Here's how the part is built. I have some questions about the finished solid (model axes, mm). A direction names the side the tool comes from. Coordinates: 2 decimals unless noted, no trailing zeros. Write each loop counter-clockwise with the first axis right and the second up, starting at its lowest first coordinate (ties: lowest second). Pieces come first, ordered by that corner, then holes.
from build123d import *

# Parameters (mm, degrees)
SKETCH1_R                = 13.7
BOSS_EXTRUDE1_DEPTH      = 101
SKETCH5_W                = 55.5
SKETCH5_H                = 56.561345004
BOSS_EXTRUDE2_DEPTH      = 2.6
CUT_EXTRUDE4_DEPTH       = 2.6
BOSS_EXTRUDE4_DEPTH      = 6
SKETCH8_W                = 33.3
SKETCH8_H                = 11.7
BOSS_EXTRUDE5_DEPTH      = 2.8
SKETCH9_W                = 33.3
SKETCH9_H                = 2.7
BOSS_EXTRUDE6_DEPTH      = 22.2
FILLET2_R                = 5
REVOLVE1_ANGLE           = 40
REVOLVE1_OTHER_WAY_ANGLE = 40
FILLET6_R                = 9


with BuildPart() as part:
    # Sketch1 → Boss-Extrude1 (new body)
    with BuildSketch(Plane.XY):
        with Locations(Location((0, 0, 0), (0, 0, 180))):
            Circle(SKETCH1_R)
    extrude(amount=BOSS_EXTRUDE1_DEPTH)

    # Sketch5 → Boss-Extrude2 (add)
    with BuildSketch(Plane(origin=(0, 0, 0), x_dir=(-1, 0, 0), z_dir=(0, 0, -1))):
        Rectangle(SKETCH5_W, SKETCH5_H)
    extrude(amount=BOSS_EXTRUDE2_DEPTH)

    # Sketch6 → Cut-Extrude4 (cut)
    with BuildSketch(Plane(origin=(0, 0, -2.6), x_dir=(-1, 0, 0), z_dir=(0, 0, -1))):
        Polygon((27.75, 28.280672502), (18.35, 28.280672502), (27.75, 16.680672502), align=None)
        Polygon((-16.15, -28.280672502), (-27.75, -16.680672502), (-27.75, -28.280672502), align=None)
        Polygon((27.75, -18.880672502), (18.35, -28.280672502), (27.75, -28.280672502), align=None)
        Polygon((-27.75, 16.680672502), (-27.75, 28.280672502), (-16.15, 28.280672502), align=None)
    extrude(amount=-CUT_EXTRUDE4_DEPTH, mode=Mode.SUBTRACT)

    # Sketch7 → Boss-Extrude4 (add)
    with BuildSketch(Plane(origin=(0, 0, -2.6), x_dir=(-1, 0, 0), z_dir=(0, 0, -1))):
        Polygon((1.1, 25.680672502), (16.366645995, 25.680672502), (16.366645995, 22.680672502), (-16.933354005, 22.680672502), (-16.933354005, 25.680672502), align=None)
    extrude(amount=BOSS_EXTRUDE4_DEPTH)

    # Sketch8 → Boss-Extrude5 (add)
    with BuildSketch(Plane(origin=(0, 0, -8.6), x_dir=(-1, 0, 0), z_dir=(0, 0, -1))):
        with Locations((-0.283354005, 19.830672502)):
            Rectangle(SKETCH8_W, SKETCH8_H)
    extrude(amount=BOSS_EXTRUDE5_DEPTH)

    # Sketch9 → Boss-Extrude6 (add)
    with BuildSketch(Plane(origin=(0, 25.680672502, 0), x_dir=(1, 0, 0), z_dir=(0, 1, 0))):
        with Locations((0.283354005, 10.05)):
            Rectangle(SKETCH9_W, SKETCH9_H)
    extrude(amount=BOSS_EXTRUDE6_DEPTH)

    # Fillet2
    # the kernel refuses this fillet: 5 mm, written as the material it adds along each edge
    with BuildSketch(Plane(origin=(-16.366645995, 25.680672502, -2.6), x_dir=(0, 1, 0), z_dir=(1, 0, 0))) as fillet2_piece_1_section:
        with BuildLine():
            CenterArc((5, -4.38634244), FILLET2_R, 118.685402014, 61.314597986)
            Line((0, -4.38634244), (-0.1, -4.38634244))
            Line((-0.1, -4.38634244), (-0.1, 0))
            Line((-0.1, 0), (0, 0.1))
            ThreePointArc((0, 0.1), (1.3, 0.1), (2.552, 0.087726849))
            Line((2.552, 0.087726849), (2.6, 0))
        make_face()
    fillet2_piece_1 = extrude(amount=33.3, mode=Mode.PRIVATE)
    fillet2_piece_1 = split(fillet2_piece_1, bisect_by=Plane(origin=(9.175527955, 35.255144547, -3.690317045), z_dir=(-0.7071067811865442, -0.7071067811865509, 0)), keep=Keep.TOP, mode=Mode.PRIVATE)
    add(fillet2_piece_1)
    with BuildSketch(Plane(origin=(-16.366645995, 22.680672502, -2.6), x_dir=(0, -1, 0), z_dir=(1, 0, 0))) as fillet2_piece_2:
        with BuildLine():
            CenterArc((FILLET2_R, FILLET2_R), FILLET2_R, 180, 90)
            Line((0, FILLET2_R), (-FILLET2_R * 0.02, FILLET2_R))
            Line((-FILLET2_R * 0.02, FILLET2_R), (-FILLET2_R * 0.02, -FILLET2_R * 0.02))
            Line((-FILLET2_R * 0.02, -FILLET2_R * 0.02), (FILLET2_R, -FILLET2_R * 0.02))
            Line((FILLET2_R, -FILLET2_R * 0.02), (FILLET2_R, 0))
        make_face()
    extrude(amount=33.3)
    with BuildSketch(Plane(origin=(-16.366645995, 22.680672502, -8.6), x_dir=(0, -1, 0), z_dir=(1, 0, 0)), Plane(origin=(16.933354005, 25.680672502, -8.7), x_dir=(0, 1, 0), z_dir=(-1, 0, 0))) as fillet2_piece_3:
        with BuildLine():
            CenterArc((FILLET2_R, -FILLET2_R), FILLET2_R, 90, 90)
            Line((0, -FILLET2_R), (-FILLET2_R * 0.02, -FILLET2_R))
            Line((-FILLET2_R * 0.02, -FILLET2_R), (-FILLET2_R * 0.02, FILLET2_R * 0.02))
            Line((-FILLET2_R * 0.02, FILLET2_R * 0.02), (FILLET2_R, FILLET2_R * 0.02))
            Line((FILLET2_R, FILLET2_R * 0.02), (FILLET2_R, 0))
        make_face()
    extrude(amount=33.3)

    # Sketch10 → Revolve1 (revolve)
    with BuildSketch(Plane.ZY):
        with BuildLine():
            Line((101, 13.7), (101, 16))
            ThreePointArc((101, 16), (99.554707727, 16.71784268), (98.02630764, 16.2))
            ThreePointArc((98.02630764, 16.2), (94.964280854, 14.479645567), (91.539696179, 13.7))
            Line((91.539696179, 13.7), (101, 13.7))
        make_face()
    revolve(axis=Axis((0, 0, 101.100764075), (0, 0, -1)), revolution_arc=REVOLVE1_ANGLE)

    # Sketch10 → Revolve1 other way (revolve)
    with BuildSketch(Plane.ZY):
        with BuildLine():
            Line((101, 13.7), (101, 16))
            ThreePointArc((101, 16), (99.554707727, 16.71784268), (98.02630764, 16.2))
            ThreePointArc((98.02630764, 16.2), (94.964280854, 14.479645567), (91.539696179, 13.7))
            Line((91.539696179, 13.7), (101, 13.7))
        make_face()
    revolve(axis=Axis((0, 0, 101.100764075), (0, 0, 1)), revolution_arc=REVOLVE1_OTHER_WAY_ANGLE)

    # Fillet6
    fillet6_edges = [part.edges().sort_by_distance(p)[0] for p in [
        (13.7, 0, 0),
    ]]
    fillet(fillet6_edges, radius=FILLET6_R)


solid = part.part
1. I want a section at B-B (y = 0). List the corners of the cut face in (x, z) for me.
2. For pin 1 Ø5 at (y, z) = (-15, 21) entering from -X; pin 2 Ø1.5 at (x, y) = (19, -7) entering from -Z; pin 3 Ø4 at (x, y) = (6.5, 16.5) entering from +Z; pin 4 Ø3 at (x, z) = (-7.5, -10) entering from -Y, each with a flat end and sliding along its axis, tell me the tip position at first contact or that it passes through.
3. Thinking about a two-plate mould opening in Z: for faces 4 (the face through (0, 39, -8.7)), 5 (the face through (0.05, 26.88, -3.74)), 6 (the face through (-27.75, -1, -1)), which applies, pulls with the +Z half, pulls with the -Z half, needs draft (parallel to the pull), parting line crosses it, or undercut?
4. On a 3-axis mill with a long thin cutter (end or side, diameter ignored), from which of +Z, -Z, +X, -X, +Y, -Y can I reach the whole of each face in a straight line? I mean faces 1 (the face through (-9.575, 11.411, 98.306)), 2 (the face through (0.05, 20.453, -3.439)), 3 (the face through (19, 13, 0)). Say none if no direction works.
5. I want a section at C-C (z = 38.5). List the corners of the cut face in (x, y) for me, then the cut area to 3 significant figures.
6. If I drill on line 1 (Z direction, x = 6, y = 42); line 2 (X direction, y = 0.5, z = 66); line 3 (Z direction, x = 10, y = 12), over which ranges is the centre line in solid material (lowest first)?
7. I want a section at D-D (y = 39). List the corners of the cut face in (x, z) for me, then the cut area to 3 significant figures.
8. I want a section at A-A (x = 0). List the corners of the cut face in (y, z) for me.
Response values:
1. outline: (-27.75, -2.6) - (27.75, -2.6) - (27.75, 0) - (22.7, 0) arc R9 cw to (13.7, 9) - (13.7, 101) - (-13.7, 101) - (-13.7, 9) arc R9 cw to (-22.7, 0) - (-27.75, 0) - close
2. pin 1: stops at x = -5.61
2. pin 2: stops at z = -2.6
2. pin 3: stops at z = 101
2. pin 4: stops at y = 13.98
3. face 4: pulls with the +Z half
3. face 5: undercut
3. face 6: needs draft
4. face 1: +Z, -X
4. face 2: +X, -X, -Y
4. face 3: +Z
5. outline: circle Ø27.4 at (0, 0)
5. area: 590 mm2
6. line 1: z = -11.4 to -8.7
6. line 2: x = -13.69 to 13.69
6. line 3: z = -2.6 to 3.44, 97.21 to 101
7. outline: (-16.37, -11.4) - (16.93, -11.4) - (16.93, -8.7) - (-16.37, -8.7) - close
7. area: 89.9 mm2
8. outline: (-28.28, -2.6) - (17.68, -2.6) arc R5 cw to (22.26, -5.6) arc R5 cw to (17.68, -8.6) - (13.98, -8.6) - (13.98, -11.4) - (47.88, -11.4) - (47.88, -8.7) - (30.68, -8.7) arc R5 cw to (25.96, -5.34) arc R5 cw to (28.28, -2.6) - (28.28, 0) - (22.7, 0) arc R9 cw to (13.7, 9) - (13.7, 91.54) arc R12.24 cw to (16.2, 98.03) arc R2.1 ccw to (16, 101) - (-13.7, 101) - (-13.7, 9) arc R9 cw to (-22.7, 0) - (-28.28, 0) - close
